Part print with two shaded views. Sizes in mm from the minimum x, y, z corner. A direction names the side the tool comes from. Round coordinates to 2 decimals unless told otherwise and drop trailing zeros. Loops run counter-clockwise (first coordinate to the right, second up) from the corner with the lowest first, then second, coordinate; pieces in that order, holes last. Notation, with made-up numbers: (48, 60) -> (87, 60) arc R18 ccw to (87, 89) -> close; hole circle Ø4 at (15.5, 50.5). An arc over 180 degrees is marked (long way). Answer as a JSON object with one key per item and string values. Group by question number.
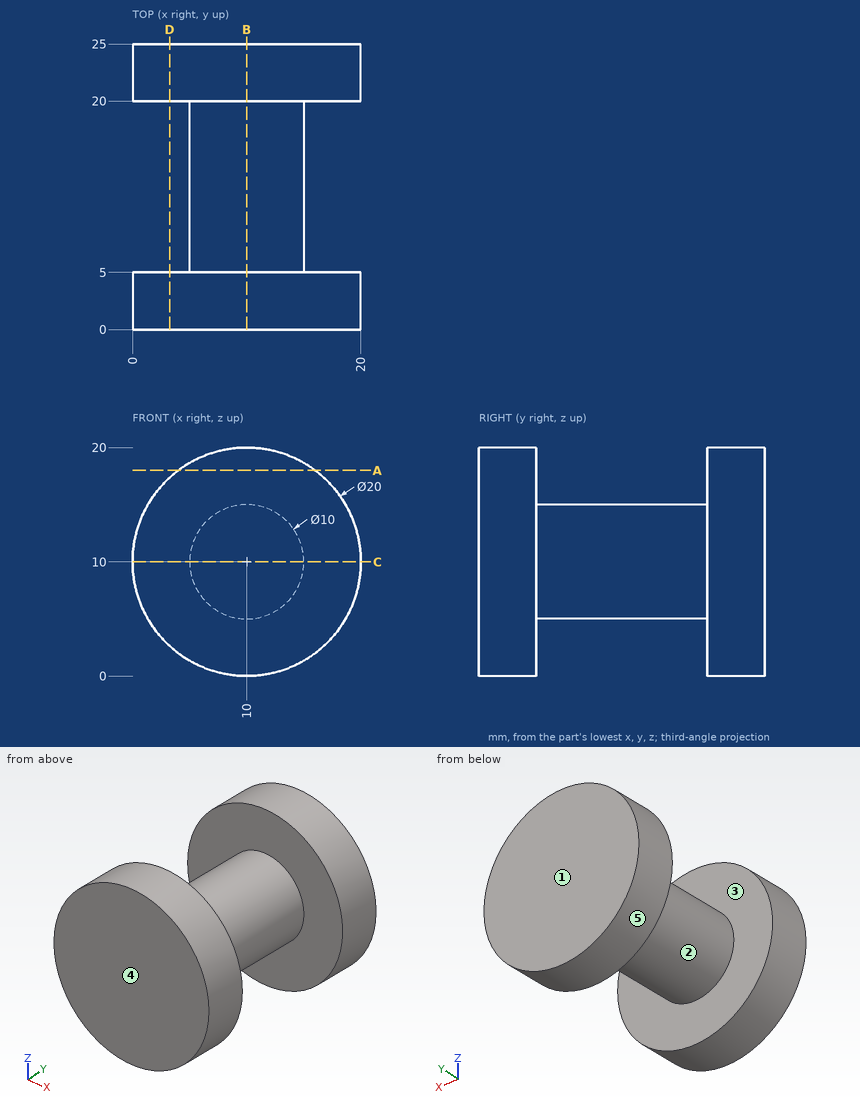
Item 1: Band-saw the part on B-B, the plane x = 10. List the corners of the cut face in (y, z).
Item 2: Band-saw the part on A-A, the plane z = 18. List the corners of the cut face in (x, y), plus the area to 3 significant figures.
Item 3: Two-plate mould, pull along Y, no slides. Class the marked faces 3, 4 and 5: pulls with the +Y half, pulls with the -Y half, needs draft (parallel to the pull), parting line crosses it, or undercut.
Item 4: Which spindle directions (+Z, -Z, +X, -X, +Y, -Y) get a long thin tool onto all of the face, cutting with end or side? Do the marked faces 1 and 2. Say none if no direction does.
Item 5: Drill centre lines: line 1 (Y direction, x = 18.5, z = 14.25); line 2 (X direction, y = 22.75, z = 12); line 3 (X direction, y = 20.25, z = 1.25). Where is each one in solid material? Low to high.
Item 6: Drop a flat-ended pin along its axis: pin 1 Ø1 at (x, y) = (5.5, 13) entering from +Z. Give the stop position or say it passes through.
Item 7: Band-saw the part on C-C, the plane z = 10. List the corners of the cut face in (x, y).
Item 8: Band-saw the part on D-D, the plane x = 3.25. List the corners of the cut face in (y, z).
Entries:
{
 "1": {"outline": "(0, 0) -> (5, 0) -> (5, 5) -> (20, 5) -> (20, 0) -> (25, 0) -> (25, 20) -> (20, 20) -> (20, 15) -> (5, 15) -> (5, 20) -> (0, 20) -> close"},
 "2": {"outline": "(4, 0) -> (16, 0) -> (16, 5) -> (4, 5) -> close; (4, 20) -> (16, 20) -> (16, 25) -> (4, 25) -> close", "area": "120 mm²"},
 "3": {"face 3": "undercut", "face 4": "pulls with the -Y half", "face 5": "needs draft"},
 "4": {"face 1": "+Z, -Z, +X, -X, +Y", "face 2": "none"},
 "5": {"line 1": "0 to 5, 20 to 25", "line 2": "0.2 to 19.8", "line 3": "5.16 to 14.84"},
 "6": {"pin 1": "z = 13"},
 "7": {"outline": "(0, 0) -> (20, 0) -> (20, 5) -> (15, 5) -> (15, 20) -> (20, 20) -> (20, 25) -> (0, 25) -> (0, 20) -> (5, 20) -> (5, 5) -> (0, 5) -> close"},
 "8": {"outline": "(0, 2.62) -> (5, 2.62) -> (5, 17.38) -> (0, 17.38) -> close; (20, 2.62) -> (25, 2.62) -> (25, 17.38) -> (20, 17.38) -> close"}
}
